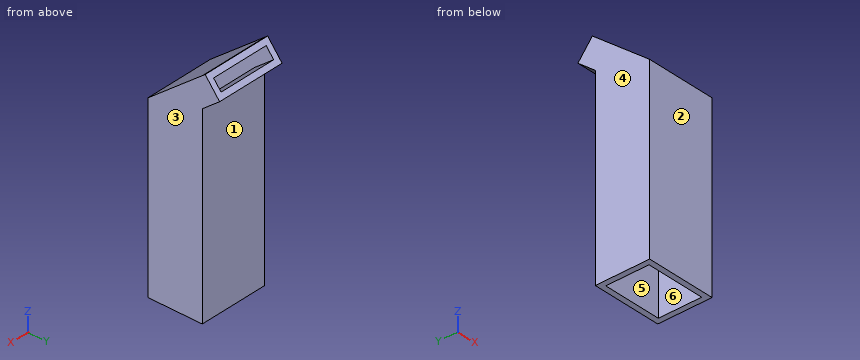
```python
from build123d import *

# Parameters (mm, degrees)
F0_W      = 19
F0_H      = 14.7
F0_W_2    = 17
F0_H_2    = 12.7
F1_DEPTH  = 40
F3_DEPTH  = 19.001
F5_DEPTH  = 19
F6_T      = -1.5
F8_DEPTH  = 19.001
F9_W      = 19
F9_H      = 14.7
F9_W_2    = 16
F9_H_2    = 11.7
F10_DEPTH = 20


with BuildPart() as f1:
    # F0 (on Top) → F1 (new body)
    with BuildSketch(Plane.XY):
        with Locations((-8.5, 6.35)):
            Rectangle(F0_W, F0_H)
        with Locations((-8.5, 6.35)):
            Rectangle(F0_W_2, F0_H_2, mode=Mode.SUBTRACT)
        with Locations((-8.5, 6.35)):
            Rectangle(F0_W_2, F0_H_2)
    extrude(amount=F1_DEPTH)

    # F2 (on face) → F3 (cut, through all)
    with BuildSketch(Plane.YZ.offset(1)):
        Polygon((-1, 40), (-1, 28.249386698), (13.7, 40), align=None)
    extrude(amount=-F3_DEPTH, mode=Mode.SUBTRACT)

    # F4 (on face) → F5 (join)
    with BuildSketch(Plane.YZ.offset(1)):
        Polygon((18.3866723446, 43.7463451969), (13.7, 40), (13.7, 32), (18.3866723446, 35.7463451969), align=None)
    extrude(amount=-F5_DEPTH)

    # F6
    f6_openings = [f1.faces().sort_by_distance(p)[0] for p in [
        (-8.5, 18.386672, 39.746345),
        (-8.5, 6.35, 0),
    ]]
    offset(amount=F6_T, openings=f6_openings, kind=Kind.INTERSECTION)

    # F7 (on face) → F8 (cut, through all)
    with BuildSketch(Plane(origin=(-18, 0, 0), x_dir=(0, -1, 0), z_dir=(-1, 0, 0))):
        Polygon((-18.3866723446, 43.7463451969), (-18.3866723446, 35.7463451969), (-14.4849184718, 40.627433567), align=None)
    extrude(amount=-F8_DEPTH, mode=Mode.SUBTRACT)

    # F9 (on face) → F10 (join)
    with BuildSketch(Plane(origin=(0, 0, 0), x_dir=(1, 0, 0), z_dir=(0, 0, -1))):
        with Locations((-8.5, -6.35)):
            Rectangle(F9_W, F9_H)
        with Locations((-8.5, -6.35)):
            Rectangle(F9_W_2, F9_H_2, mode=Mode.SUBTRACT)
    extrude(amount=F10_DEPTH)


solid = f1.part
```
CAD build for the part. Positions are in the model's coordinates, mm. Face numbers are marked on the shaded views. A direction names the side the tool comes from. Round coordinates to 2 decimals unless told otherwise and drop trailing zeros. Order: outer loops, then holes, each group sorted by start corner. A loop starts at its lowest first (then second) coordinate and runs counter-clockwise, first axis right, second up.
Item 1: Saw through at B-B on z = -4. Write the cut outline in (x, y).
Item 2: Saw through at A-A on x = -8.5. Write the cut outline in (y, z), then the cut area to 3 significant figures.
Item 3: Probe line 1 along X through (y, z) = (8.25, 1.5); line 2 along Y through (x, z) = (-6.5, 13); line 3 along Y through (x, z) = (-16.75, 19). List the from-to ranges inside material, lowest first.
Item 4: Mould opens along X. For the marked faces 3, 4, 5 and 6 say: pulls with the +X half, pulls with the -X half, needs draft (parallel to the pull), parting line crosses it, or undercut.
Item 5: Tool access for the marked faces 1 and 2: list every direction of +Z, -Z, +X, -X, +Y, -Y with a clear straight run to the whole face (end or side of a thin tool).
Item 6: Pin check, flat tips, straight feed: pin 1 (10 mm diameter, centred on x = -9, z = -5, fed in from +Y); pin 2 (6 mm diameter, centred on x = -9, y = 8, fed in from -Z); pin 3 (1.5 mm diameter, centred on x = -3.5, z = 32, fed in from -Y). Stop position of each tip, or through.
Item 7: Saw through at C-C on y = 10.75. Write the cut outline in (x, z).
Item 8: Saw through at D-D on z = 35. Write the cut outline in (x, y) (3 decimals).
Reported:
1. outline: (-18, -1) - (1, -1) - (1, 13.7) - (-18, 13.7) - close; hole (-16.5, 0.5) - (-0.5, 0.5) - (-0.5, 12.2) - (-16.5, 12.2) - close
2. outline: (-1, -20) - (0.5, -20) - (0.5, 27.53) - (15.42, 39.46) - (14.48, 40.63) - (-1, 28.25) - close; (12.2, -20) - (13.7, -20) - (13.7, 32) - (18.39, 35.75) - (17.45, 36.92) - (12.2, 32.72) - close
2. area: 189 mm2
3. line 1: x = -18 to -16.5, -0.5 to 1
3. line 2: y = -1 to 0.5, 12.2 to 13.7
3. line 3: y = -1 to 13.7
4. face 3: pulls with the +X half
4. face 4: pulls with the -X half
4. face 5: undercut
4. face 6: undercut
5. face 1: -Z, +X, -X, +Y
5. face 2: +Z, -Z, +X, -X, -Y
6. pin 1: stops at y = 13.7
6. pin 2: stops at z = 31.13
6. pin 3: stops at y = 2.75
7. outline: (-18, -20) - (-16.5, -20) - (-16.5, 35.72) - (-0.5, 35.72) - (-0.5, -20) - (1, -20) - (1, 37.64) - (-18, 37.64) - close
8. outline: (-18, 7.445) - (1, 7.445) - (1, 17.453) - (-18, 17.453) - close; hole (-16.5, 9.847) - (-0.5, 9.847) - (-0.5, 15.051) - (-16.5, 15.051) - close
